```python
from build123d import *

# Parameters (mm, degrees)
SKETCH2_R           = 1
BOSS_EXTRUDE1_DEPTH = 3
SKETCH3_W           = 3.515258844
SKETCH3_H           = 10
BOSS_EXTRUDE2_DEPTH = 2
CHAMFER1_SIZE       = 2
FILLET1_R           = 4
FILLET2_R           = 1


with BuildPart() as part:
    # Sketch2 → Boss-Extrude1 (new body)
    with BuildSketch(Plane.XY):
        with BuildLine():
            Line((47.48595993, 0.792979965), (51.48595993, 0.792979965))
            Line((51.48595993, 0.792979965), (51.48595993, 10.942979965))
            Line((51.48595993, 10.942979965), (17.68595993, 10.942979965))
            Line((17.68595993, 10.942979965), (17.68595993, 0.792979965))
            Line((17.68595993, 0.792979965), (24.68595993, 0.792979965))
            Line((24.68595993, 0.792979965), (24.68595993, 6.292979965))
            ThreePointArc((24.68595993, 6.292979965), (24.33240654, 7.146533356), (25.18595993, 6.792979965))
            Line((25.18595993, 6.792979965), (46.98595993, 6.792979965))
            ThreePointArc((46.98595993, 6.792979965), (47.839513321, 7.146533356), (47.48595993, 6.292979965))
            Line((47.48595993, 6.292979965), (47.48595993, 0.792979965))
        make_face()
        with Locations((44.48595993, 8.942979965)):
            Circle(SKETCH2_R, mode=Mode.SUBTRACT)
        with Locations((21.68595993, 8.942979965)):
            Circle(SKETCH2_R, mode=Mode.SUBTRACT)
    extrude(amount=BOSS_EXTRUDE1_DEPTH)

    # Mirror1: part across plane


with BuildPart() as part_1:
    add(part.part)
    add(part.part.mirror(Plane(origin=(0, 0.792979965, 3), x_dir=(0, 0, 1), z_dir=(0, -1, 0))))

    # Sketch3 → Boss-Extrude2 (add)
    with BuildSketch(Plane.XY.offset(3)):
        with Locations((21.943589352, 0.792979965)):
            Rectangle(SKETCH3_W, SKETCH3_H)
    extrude(amount=BOSS_EXTRUDE2_DEPTH)

    # Chamfer1
    chamfer1_edges = [part_1.edges().sort_by_distance(p)[0] for p in [
        (23.701218774, 0.792979965, 5),
    ]]
    chamfer(chamfer1_edges, length=CHAMFER1_SIZE - 0.0001)  # a hair under: the kernel refuses the full size

    # Fillet1
    fillet1_edges = [part_1.edges().sort_by_distance(p)[0] for p in [
        (51.48595993, 10.942979965, 1.5),
        (51.48595993, -9.357020035, 1.5),
    ]]
    fillet(fillet1_edges, radius=FILLET1_R)

    # Fillet2
    fillet2_edges = [part_1.edges().sort_by_distance(p)[0] for p in [
        (17.68595993, 10.942979965, 1.5),
        (17.68595993, -9.357020035, 1.5),
    ]]
    fillet(fillet2_edges, radius=FILLET2_R)


solid = part_1.part
```
Work out the finished part from the listing and answer in its coordinate system (mm). A direction names the side the tool comes from. Round coordinates to 2 decimals unless told otherwise and drop trailing zeros. Loops run counter-clockwise (first coordinate to the right, second up) from the corner with the lowest first, then second, coordinate; pieces in that order, holes last. Notation, with made-up numbers: (-34, 32) -> (-18, 32) arc R30 ccw to (-18, 65) -> close; hole circle Ø4 at (-23, 7). An arc over 180 degrees is marked (long way). Write each question's results on one line, items separated by ' | '. Start each with the question number.
1. A tool of negligible diameter and unlimited length cuts with its end or side. For faces 4 (the face through (21, 1, 5)), 5 (the face through (20.186, 1, 4)), 6 (the face through (24.686, 1, 1)), from which of +Z, -Z, +X, -X, +Y, -Y can it reach the whole face along a straight path? Write none if from no direction.
2. Find the intervals of material crossed by probe 1 along X at (y, z) = (-5.25, 0.5); probe 2 along X at (y, z) = (2.5, 2.6); probe 3 along X at (y, z) = (-5.5, 0.7), in increasing order. Write a range as from..to.
3. Given pin 1 Ø6 at (x, y) = (48, -3) entering from -Z; pin 2 Ø2.5 at (x, y) = (21.69, 8.94) entering from +Z; pin 3 Ø0.6 at (x, z) = (21, 4) entering from +Y; pin 4 Ø0.6 at (x, z) = (21.5, 4) entering from -Y, each flat-ended and moving along its own axis, determine where each tip first touches the part or whether it passes through.
4. For a pull along Y with two mould halves and no side action, classify faces 1 (the face through (34, 7, 3)), 2 (the face through (24.32, -5.55, 1.48)), 3 (the face through (22, -4.207, 4)) as +Y half, -Y half, draft (parallel to the pull), parting line (faces both ways), or undercut.
5. Section A-A (x = 32) is taken. Determine the outline of the cut face in (y, z).
6. Section C-C (z = 1.4) is taken. Determine the outline of the cut face in (x, y), plus the area to 3 significant figures.
7. Section D-D (x = 45) is taken. Determine the outline of the cut face in (y, z).
Evaluation:
1) face 4: +Z, +X, -X, +Y, -Y | face 5: +Z, -X, +Y, -Y | face 6: +Z, -Z
2) probe 1: x = 17.69..24.19, 25.18..46.99, 47.98..51.49 | probe 2: x = 17.69..24.69, 47.49..51.49 | probe 3: x = 17.69..24.28, 25.09..47.08, 47.89..51.48
3) pin 1: stops at z = 0 | pin 2: stops at z = 3 | pin 3: stops at y = 5.79 | pin 4: stops at y = -4.21
4) face 1: draft | face 2: undercut | face 3: -Y half
5) outline: (-9.36, 0) -> (-5.21, 0) -> (-5.21, 3) -> (-9.36, 3) -> close; (6.79, 0) -> (10.94, 0) -> (10.94, 3) -> (6.79, 3) -> close
6) outline: (17.69, -8.36) arc R1 ccw to (18.69, -9.36) -> (47.49, -9.36) arc R4 ccw to (51.49, -5.36) -> (51.49, 6.94) arc R4 ccw to (47.49, 10.94) -> (18.69, 10.94) arc R1 ccw to (17.69, 9.94) -> close; hole circle Ø2 at (21.69, -7.36); hole circle Ø2 at (21.69, 8.94); hole (24.69, -4.71) arc R0.5 ccw (long way) to (25.19, -5.21) -> (46.99, -5.21) arc R0.5 ccw (long way) to (47.49, -4.71) -> (47.49, 6.29) arc R0.5 ccw (long way) to (46.99, 6.79) -> (25.19, 6.79) arc R0.5 ccw (long way) to (24.69, 6.29) -> close; hole circle Ø2 at (44.49, -7.36); hole circle Ø2 at (44.49, 8.94) | area: 390 mm2
7) outline: (-9.36, 0) -> (-8.21, 0) -> (-8.21, 3) -> (-9.36, 3) -> close; (-6.5, 0) -> (-5.21, 0) -> (-5.21, 3) -> (-6.5, 3) -> close; (6.79, 0) -> (8.09, 0) -> (8.09, 3) -> (6.79, 3) -> close; (9.8, 0) -> (10.94, 0) -> (10.94, 3) -> (9.8, 3) -> close
